from build123d import *

# Parameters (mm, degrees)
SKETCH1_R           = 3
BOSS_EXTRUDE1_DEPTH = 2


with BuildPart() as part:
    # Sketch1 → Boss-Extrude1 (new body)
    with BuildSketch(Plane.XY):
        with BuildLine():
            Line((-3.7366, 240), (-3.7366, 0))
            ThreePointArc((-3.7366, 0), (-2.642175199, -2.642175199), (0, -3.7366))
            Line((0, -3.7366), (290, -3.7366))
            ThreePointArc((290, -3.7366), (292.642175199, -2.642175199), (293.7366, 0))
            Line((293.7366, 0), (293.7366, 240))
            ThreePointArc((293.7366, 240), (292.642175199, 242.642175199), (290, 243.7366))
            Line((290, 243.7366), (0, 243.7366))
            ThreePointArc((0, 243.7366), (-2.642175199, 242.642175199), (-3.7366, 240))
        make_face()
        with Locations((284.7366, 5.2634)):
            Circle(SKETCH1_R, mode=Mode.SUBTRACT)
        with Locations((284.7366, 234.7366)):
            Circle(SKETCH1_R, mode=Mode.SUBTRACT)
        with Locations((5.2634, 234.7366)):
            Circle(SKETCH1_R, mode=Mode.SUBTRACT)
        with Locations((5.2634, 5.2634)):
            Circle(SKETCH1_R, mode=Mode.SUBTRACT)
        with BuildLine():
            Line((278.7366, -0.7366), (11.2634, -0.7366))
            Line((11.2634, -0.7366), (11.2634, 5.2634))
            ThreePointArc((11.2634, 5.2634), (9.506040687, 9.506040687), (5.2634, 11.2634))
            Line((5.2634, 11.2634), (-0.7366, 11.2634))
            Line((-0.7366, 11.2634), (-0.7366, 228.7366))
            Line((-0.7366, 228.7366), (5.2634, 228.7366))
            ThreePointArc((5.2634, 228.7366), (9.506040687, 230.493959313), (11.2634, 234.7366))
            Line((11.2634, 234.7366), (11.2634, 240.7366))
            Line((11.2634, 240.7366), (278.7366, 240.7366))
            Line((278.7366, 240.7366), (278.7366, 234.7366))
            ThreePointArc((278.7366, 234.7366), (280.493959313, 230.493959313), (284.7366, 228.7366))
            Line((284.7366, 228.7366), (290.7366, 228.7366))
            Line((290.7366, 228.7366), (290.7366, 11.2634))
            Line((290.7366, 11.2634), (284.7366, 11.2634))
            ThreePointArc((284.7366, 11.2634), (280.493959313, 9.506040687), (278.7366, 5.2634))
            Line((278.7366, 5.2634), (278.7366, -0.7366))
        make_face(mode=Mode.SUBTRACT)
    extrude(amount=BOSS_EXTRUDE1_DEPTH)


solid = part.part
Build history of the part. All positions in model axes, mm. Round coordinates to 2 decimals unless told otherwise and drop trailing zeros. Loops run counter-clockwise (first coordinate to the right, second up) from the corner with the lowest first, then second, coordinate; pieces in that order, holes last. Notation, with made-up numbers: (0.25, 16) -> (14.25, 16) arc R18 cw to (14.25, 28) -> close; hole circle Ø11 at (57.5, 64). An arc over 180 degrees is marked (long way). Answer in a Markdown table with one row per item.
Item 1: Pin check, flat tip, straight feed: pin 1 (5 mm diameter, centred on x = 5.26, y = 5.26, fed in from -Z). Stop position of the tip, or through.
Answers below:
| item | result |
|---|---|
| pin 1 | passes through |
Item 2: Drill centre lines: L1, parallel to X at y = 129.5, z = 1.25; L2, parallel to Y at x = 66.5, z = 0.85; L3, parallel to X at y = 7, z = 1.85. Where is each one in solid material? Low to high. Write a range as [from, to].
Answers below:
| item | result |
|---|---|
| L1 | x = [-3.74, -0.74], [290.74, 293.74] |
| L2 | y = [-3.74, -0.74], [240.74, 243.74] |
| L3 | x = [-3.74, 2.82], [7.71, 11.01], [278.99, 282.29], [287.18, 293.74] |
Item 3: Saw through at A-A (y = 119). Write the cut outline in (x, z).
Answers below:
| item | result |
|---|---|
| outline | (-3.74, 0) -> (-0.74, 0) -> (-0.74, 2) -> (-3.74, 2) -> close; (290.74, 0) -> (293.74, 0) -> (293.74, 2) -> (290.74, 2) -> close |
Item 4: Saw through at B-B (x = 44). Write the cut outline in (y, z).
Answers below:
| item | result |
|---|---|
| outline | (-3.74, 0) -> (-0.74, 0) -> (-0.74, 2) -> (-3.74, 2) -> close; (240.74, 0) -> (243.74, 0) -> (243.74, 2) -> (240.74, 2) -> close |
Item 5: Saw through at C-C (z = 1.25). Write the cut outline in (x, y).
Answers below:
| item | result |
|---|---|
| outline | (-3.74, 0) arc R3.74 ccw to (0, -3.74) -> (290, -3.74) arc R3.74 ccw to (293.74, 0) -> (293.74, 240) arc R3.74 ccw to (290, 243.74) -> (0, 243.74) arc R3.74 ccw to (-3.74, 240) -> close; hole (-0.74, 11.26) -> (5.26, 11.26) arc R6 cw to (11.26, 5.26) -> (11.26, -0.74) -> (278.74, -0.74) -> (278.74, 5.26) arc R6 cw to (284.74, 11.26) -> (290.74, 11.26) -> (290.74, 228.74) -> (284.74, 228.74) arc R6 cw to (278.74, 234.74) -> (278.74, 240.74) -> (11.26, 240.74) -> (11.26, 234.74) arc R6 cw to (5.26, 228.74) -> (-0.74, 228.74) -> close; hole circle Ø6 at (5.26, 5.26); hole circle Ø6 at (5.26, 234.74); hole circle Ø6 at (284.74, 5.26); hole circle Ø6 at (284.74, 234.74) |
